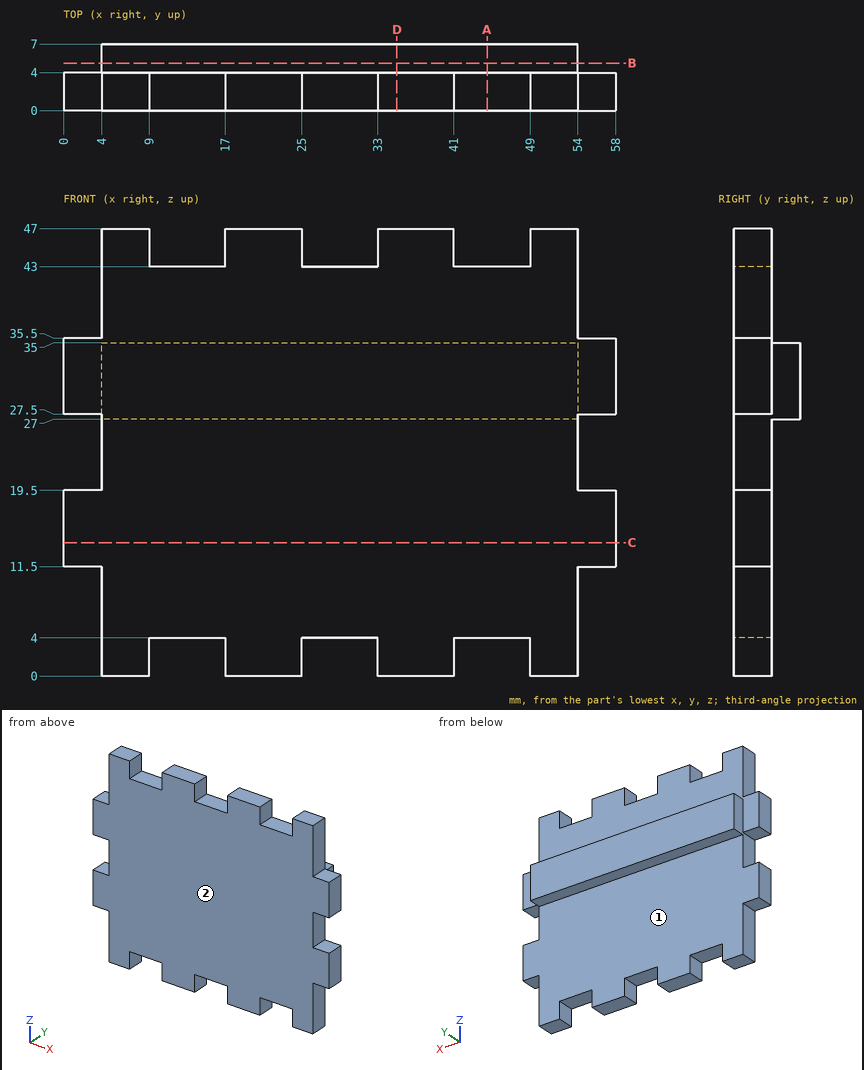
Check sheet for the drawn part. Datum: minimum x, y, z corner. Units: mm. A direction names the side the tool comes from. Coordinates: 2 decimals unless noted, no trailing zeros. Loops run counter-clockwise (first coordinate to the right, second up) from the corner with the lowest first, then second, coordinate; pieces in that order, holes last. Notation, with made-up numbers: (77, 88.25) -> (111, 88.25) arc R13 ccw to (111, 96.25) -> close; hole circle Ø5 at (67, 24.25). An arc over 180 degrees is marked (long way). Write each question's results on one line, items separated by ' | '.
Item 1: Section check D-D, the plane x = 35. Enter the section's corners in (y, z), plus the area to 3 significant figures.
Found:
outline: (0, 0) -> (4, 0) -> (4, 27) -> (7, 27) -> (7, 35) -> (4, 35) -> (4, 47) -> (0, 47) -> close | area: 212 mm2
Item 2: Section check B-B, the plane y = 5. Enter the section's corners in (x, z).
Found:
outline: (4, 27) -> (54, 27) -> (54, 35) -> (4, 35) -> close
Item 3: Gauge pin test, flat ends, axial feed: pin 1 (2 mm diameter, centred on x = 2.5, y = 3, fed in from -Z); pin 2 (2 mm diameter, centred on x = 31, z = 5.5, fed in from +Y); pin 3 (3 mm diameter, centred on x = 27, y = 1.5, fed in from +Z). Record the tip position at first contact, or that the pin passes through.
Found:
pin 1: stops at z = 11.5 | pin 2: stops at y = 4 | pin 3: stops at z = 43
Item 4: Tool access check on the marked faces 1 and 2. Record the directions out of +Z, -Z, +X, -X, +Y, -Y that give a thin tool (end or side, any length) a straight path to the whole face; none if there is none.
Found:
face 1: -Z, +X, -X, +Y | face 2: +Z, -Z, +X, -X, -Y
Item 5: Material ranges on L1, parallel to Z at x = 19.5, y = 4.25; L2, parallel to Y at x = 8.5, z = 10; L3, parallel to X at y = 4.75, z = 32, recorded low to high.
Found:
L1: z = 27 to 35 | L2: y = 0 to 4 | L3: x = 4 to 54
Item 6: Section check C-C, the plane z = 14. Enter the section's corners in (x, y).
Found:
outline: (0, 0) -> (58, 0) -> (58, 4) -> (0, 4) -> close
Item 7: Section check A-A, the plane x = 44.5. Enter the section's corners in (y, z).
Found:
outline: (0, 4) -> (4, 4) -> (4, 27) -> (7, 27) -> (7, 35) -> (4, 35) -> (4, 43) -> (0, 43) -> close
